For this review, take the finished solid that the model builds, in its own axes (mm). Face numbers are marked on the shaded views. A direction names the side the tool comes from. Coordinates: 2 decimals unless noted, no trailing zeros. Write each loop counter-clockwise with the first axis right and the second up, starting at its lowest first coordinate (ties: lowest second). Pieces come first, ordered by that corner, then holes. Notation, with made-up numbers: (68.5, 80.5) -> (83.5, 80.5) arc R24 ccw to (83.5, 106.5) -> close; hole circle Ø7 at (-23, 65.5). An arc over 180 degrees is marked (long way). One line per item, written item: value. Start each with the question number.
1) Add section B-B (y = 10.5). State the section outline as (x, z) points, and give its area (3 significant figures).
2) Add section C-C (x = -22.5). State the section outline as (y, z) points.
3) Add section A-A (z = -4). State the section outline as (x, y) points (3 decimals).
4) Machinability: for the marked faces 1, 2 and 3, which of the approach directions +Z, -Z, +X, -X, +Y, -Y give a long, thin tool a straight path to every point of the face, cutting with its end or side? Answer none if there is none.
5) For pin 1 Ø1.5 at (x, z) = (-26, 3.5) entering from -Y; pin 2 Ø4 at (x, z) = (-22, 1) entering from +Y; pin 3 Ø2 at (y, z) = (7.5, -2) entering from -X, all flat-tipped, find the tip position at first contact; note any pin that passes through.
6) For probe 1 along Y at (x, z) = (-23.5, 0.75); probe 2 along X at (y, z) = (-10.5, 2.75); probe 3 along X at (y, z) = (-11.5, 0.25), list the stretches that pass through material, from the lowest coordinate up. Write a range as from..to.
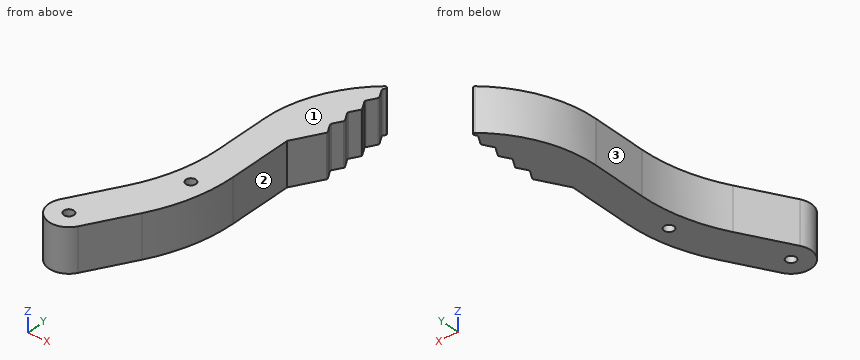
from build123d import *

# Parameters (mm, degrees)
SKETCH1_R           = 1.5
BOSS_EXTRUDE1_DEPTH = 6.5
FILLET1_R           = 0.5


with BuildPart() as part:
    # Sketch1 → Boss-Extrude1 (new body, symmetric)
    with BuildSketch(Plane.XY):
        with BuildLine():
            Line((0, 25), (-5, 16.339745962))
            Line((-5, 16.339745962), (-5, -3.282032303))
            ThreePointArc((-5, -3.282032303), (-6.703708686, -16.222984558), (-11.698729811, -28.282032303))
            Line((-11.698729811, -28.282032303), (-19.607695155, -41.980762114))
            ThreePointArc((-19.607695155, -41.980762114), (-27.803847577, -44.176914536), (-30, -35.980762114))
            Line((-30, -35.980762114), (-21.698729811, -21.602540378))
            ThreePointArc((-21.698729811, -21.602540378), (-16.703708686, -9.543492634), (-15, 3.397459622))
            Line((-15, 3.397459622), (-15, 20))
            ThreePointArc((-15, 20), (-11.041019662, 36.770509831), (0, 50))
            Line((0, 50), (-1.804219591, 46.875))
            Line((-1.804219591, 46.875), (0, 43.75))
            Line((0, 43.75), (-1.804219591, 40.625))
            Line((-1.804219591, 40.625), (0, 37.5))
            Line((0, 37.5), (-1.804219591, 34.375))
            Line((-1.804219591, 34.375), (0, 31.25))
            Line((0, 31.25), (-1.804219591, 28.125))
            Line((-1.804219591, 28.125), (0, 25))
        make_face()
        with Locations((-24.803847577, -38.980762114)):
            Circle(SKETCH1_R, mode=Mode.SUBTRACT)
        with Locations((-11.275914322, -10.99786575)):
            Circle(SKETCH1_R, mode=Mode.SUBTRACT)
    extrude(amount=BOSS_EXTRUDE1_DEPTH, both=True)

    # Fillet1
    fillet1_edges = [part.edges().sort_by_distance(p)[0] for p in [
        (0, 50, 0),
        (-1.804219591, 46.875, 0),
        (0, 43.75, 0),
        (-1.804219591, 40.625, 0),
        (0, 37.5, 0),
        (-1.804219591, 34.375, 0),
        (0, 31.25, 0),
        (-1.804219591, 28.125, 0),
        (0, 25, 0),
    ]]
    fillet(fillet1_edges, radius=FILLET1_R)


solid = part.part
Numbers:
1. outline: (-15, -6.5) -> (-5, -6.5) -> (-5, 6.5) -> (-15, 6.5) -> close
1. area: 130 mm²
2. outline: (-44.52, -6.5) -> (-22.99, -6.5) -> (-22.99, 6.5) -> (-44.52, 6.5) -> close
3. outline: (-30, -35.981) arc R6 ccw to (-19.608, -41.981) -> (-11.699, -28.282) arc R50 ccw to (-5, -3.282) -> (-5, 16.34) -> (-0.144, 24.75) arc R0.5 ccw to (-0.144, 25.25) -> (-1.66, 27.875) arc R0.5 cw to (-1.66, 28.375) -> (-0.144, 31) arc R0.5 ccw to (-0.144, 31.5) -> (-1.66, 34.125) arc R0.5 cw to (-1.66, 34.625) -> (-0.144, 37.25) arc R0.5 ccw to (-0.144, 37.75) -> (-1.66, 40.375) arc R0.5 cw to (-1.66, 40.875) -> (-0.144, 43.5) arc R0.5 ccw to (-0.144, 44) -> (-1.66, 46.625) arc R0.5 cw to (-1.66, 47.125) -> (-1.344, 47.671) arc R0.5 ccw to (-2.105, 48.299) arc R37.5 ccw to (-15, 20) -> (-15, 3.397) arc R50 cw to (-21.699, -21.603) -> close; hole circle Ø3 at (-24.804, -38.981); hole circle Ø3 at (-11.276, -10.998)
4. face 1: +Z, +X, -X, +Y, -Y
4. face 2: +Z, -Z, +X, -Y
4. face 3: +Z, -Z, -X, +Y
5. pin 1: y = -44.96
5. pin 2: y = -18.4
5. pin 3: x = -15
6. probe 1: -44.84..-39.72, -38.24..-24.72
6. probe 2: -16.97..-12.69, -9.86..-5.52
6. probe 3: -17.27..-12.69, -9.86..-5.68
